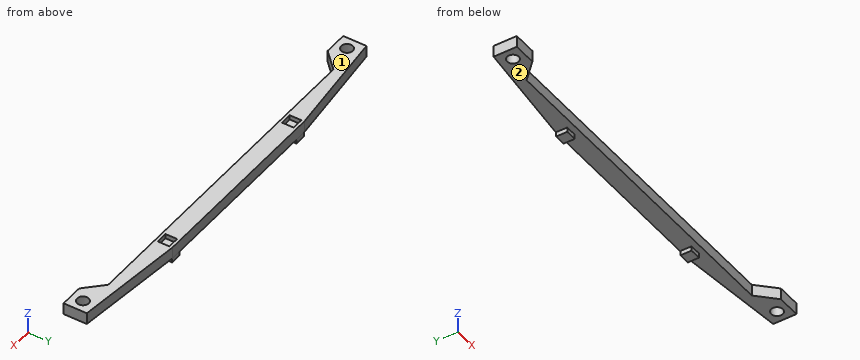
```python
from build123d import *

# Parameters (mm, degrees)
SKETCH2_W           = 180
SKETCH2_H           = 10
SKETCH2_R           = 2.5
BOSS_EXTRUDE1_DEPTH = 2.5
SKETCH3_W           = 5
SKETCH3_H           = 5
BOSS_EXTRUDE2_DEPTH = 7
CHAMFER1_SIZE       = 5
SKETCH4_W           = 5
SKETCH4_H           = 5
SKETCH4_W_2         = 4.8
SKETCH4_H_2         = 4.8
CUT_EXTRUDE1_DEPTH  = 2
CUT_EXTRUDE2_DEPTH  = 91.824005637
BOSS_EXTRUDE3_DEPTH = 5
BOSS_EXTRUDE4_DEPTH = 5
SKETCH8_W           = 5
SKETCH8_H           = 5
CUT_EXTRUDE3_DEPTH  = 2


with BuildPart() as part:
    # Sketch2 → Boss-Extrude1 (new, symmetric)
    with BuildSketch(Plane.XY):
        Rectangle(SKETCH2_W, SKETCH2_H)
        with Locations((-85, 0)):
            Circle(SKETCH2_R, mode=Mode.SUBTRACT)
        with Locations((85, 0)):
            Circle(SKETCH2_R, mode=Mode.SUBTRACT)
    extrude(amount=BOSS_EXTRUDE1_DEPTH, both=True)

    # Sketch3 → Boss-Extrude2 (add)
    with BuildSketch(Plane.XY.offset(2.5)):
        with Locations((-40, 7.5)):
            Rectangle(SKETCH3_W, SKETCH3_H)
        with Locations((40, 7.5)):
            Rectangle(SKETCH3_W, SKETCH3_H)
    extrude(amount=-BOSS_EXTRUDE2_DEPTH)

    # Chamfer1
    chamfer1_edges = [part.edges().sort_by_distance(p)[0] for p in [
        (-37.5, 5, 0),
        (-42.5, 5, 0),
        (37.5, 5, 0),
        (42.5, 5, 0),
    ]]
    chamfer(chamfer1_edges, length=CHAMFER1_SIZE - 0.0001)  # a hair under: the kernel refuses the full size

    # Sketch4 → Cut-Extrude1 (cut)
    # profile 1 of 2: a face of its own
    with BuildSketch(Plane(origin=(0, 0, -4.5), x_dir=(-1, 0, 0), z_dir=(0, 0, -1))):
        with Locations((40, 7.5)):
            Rectangle(SKETCH4_W, SKETCH4_H)
        with Locations((40, 7.5)):
            Rectangle(SKETCH4_W_2, SKETCH4_H_2, mode=Mode.SUBTRACT)
    # profile 2 of 2: a face of its own
    with BuildSketch(Plane(origin=(0, 0, -4.5), x_dir=(-1, 0, 0), z_dir=(0, 0, -1))):
        with Locations((-40, 7.5)):
            Rectangle(SKETCH4_W, SKETCH4_H)
        with Locations((-40, 7.5)):
            Rectangle(SKETCH4_W_2, SKETCH4_H_2, mode=Mode.SUBTRACT)
    extrude(amount=-CUT_EXTRUDE1_DEPTH, mode=Mode.SUBTRACT)

    # Sketch5 → Cut-Extrude2 (cut, through all)
    with BuildSketch(Plane.XY.offset(2.5)):
        Polygon((-80, -5), (-72.5, 2.5), (72.5, 2.5), (80, -5), align=None)
    extrude(amount=-CUT_EXTRUDE2_DEPTH, mode=Mode.SUBTRACT)

    # Sketch6 → Boss-Extrude3 (add)
    with BuildSketch(Plane.XY.offset(2.5)):
        Polygon((-42.5, 10), (-90, 5), (-47.5, 5), align=None)
        Polygon((42.5, 10), (47.5, 5), (90, 5), align=None)
    extrude(amount=-BOSS_EXTRUDE3_DEPTH)

    # Sketch7 → Boss-Extrude4 (add)
    with BuildSketch(Plane.XY.offset(2.5)):
        Polygon((-37.5, 10), (37.5, 10), (32.5, 5), (-32.5, 5), align=None)
    extrude(amount=-BOSS_EXTRUDE4_DEPTH)

    # Sketch8 → Cut-Extrude3 (cut)
    with BuildSketch(Plane.XY.offset(2.5)):
        with Locations((-40, 6.25)):
            Rectangle(SKETCH8_W, SKETCH8_H)
        with Locations((40, 6.25)):
            Rectangle(SKETCH8_W, SKETCH8_H)
    extrude(amount=-CUT_EXTRUDE3_DEPTH, mode=Mode.SUBTRACT)


solid = part.part
```
For this review, take the finished solid that the model builds, in its own axes (mm). Face numbers are marked on the shaded views. Give positions to 0.01 mm unless a question says otherwise; leave off trailing zeros. Loops run counter-clockwise (first coordinate to the right, second up) from the corner with the lowest first, then second, coordinate; pieces in that order, holes last. Notation, with made-up numbers: M -36,63.5 L -16,63.5 A15 ccw -16,69.5 Z; hole C 41,67 d11. An arc over 180 degrees is marked long. One line per item, written item: value. Start each with the question number.
Q1. Clearance check with flat-ended pins moving along their axes: pin 1 Ø0.6 at (y, z) = (7, -4) entering from -X; pin 2 Ø1.5 at (x, z) = (4.5, 1) entering from -Y; pin 3 Ø1 at (x, z) = (-40.5, -3.5) entering from -Y. State where each tip first meets the part, or that it passes through.
Q2. Add section D-D (x = -54). Give the boundary of the cut face in (y, z).
Q3. Add section C-C (x = 85). Give the boundary of the cut face in (y, z), and give its area (3 significant figures).
Q4. Draft analysis for pull direction X (two halves, no side actions). For the marked faces 1 and 2, state which applies: released by +X, released by -X, zero draft, split by the parting line, or undercut.
Q5. Add section B-B (z = -1). Give the boundary of the cut face in (x, y), and give its area (3 significant figures).
Q6. For L1, parallel to X at y = 1.75, z = -1; L2, parallel to X at y = 6.75, z = -4; L3, parallel to Z at x = -74.5, y = 6, list the stretches that pass through material, from the lowest coordinate up.
Q7. Add section A-A (y = 0). Give the boundary of the cut face in (x, z).
Reply:
1. pin 1: x = -42.4
1. pin 2: y = 2.5
1. pin 3: y = 5.1
2. outline: M 2.5,-2.5 L 8.79,-2.5 L 8.79,2.5 L 2.5,2.5 Z
3. outline: M -5,-2.5 L -2.5,-2.5 L -2.5,2.5 L -5,2.5 Z; M 2.5,-2.5 L 5.53,-2.5 L 5.53,2.5 L 2.5,2.5 Z
3. area: 27.6 mm²
4. face 1: zero draft
4. face 2: undercut
5. outline: M -90,-5 L -80,-5 L -72.5,2.5 L 72.5,2.5 L 80,-5 L 90,-5 L 90,5 L 42.5,10 L -42.5,10 L -90,5 Z; hole C -85,0 d5; hole C 85,0 d5
5. area: 1,280 mm²
6. L1: -90 to -86.79, -83.21 to -73.25, 73.25 to 83.21, 86.79 to 90
6. L2: -42.4 to -37.6, 37.6 to 42.4
6. L3: -2.5 to 2.5
7. outline: M -90,-2.5 L -87.5,-2.5 L -87.5,2.5 L -90,2.5 Z; M -82.5,-2.5 L -75,-2.5 L -75,2.5 L -82.5,2.5 Z; M 75,-2.5 L 82.5,-2.5 L 82.5,2.5 L 75,2.5 Z; M 87.5,-2.5 L 90,-2.5 L 90,2.5 L 87.5,2.5 Z
